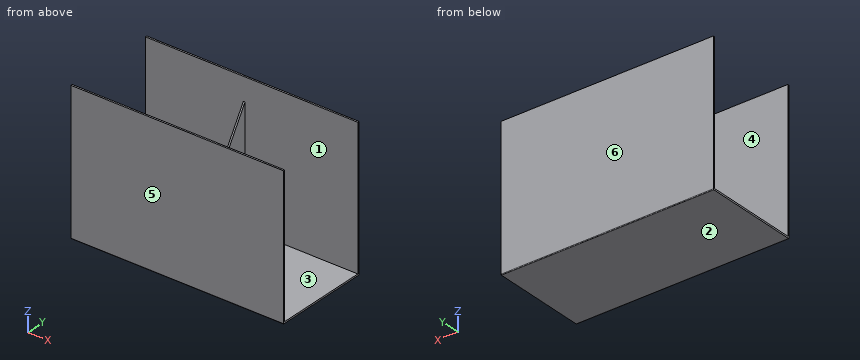
from build123d import *

# Parameters (mm, degrees)
F1_DEPTH = 650
F4_DEPTH = 5
F5_R     = 2


# Not quite as in the source:
# - a feature names something its author has since deleted; it is built from what else it names


with BuildPart() as f1:
    # F0 (on Right) → F1 (new body)
    with BuildSketch(Plane.YZ):
        Polygon((-295, 0), (0, 0), (0, 430), (-5, 430), (-5, 5), (-290, 5), (-290, 430), (-295, 430), align=None)
    extrude(amount=F1_DEPTH)

    # F3 (on offset) → F4 (join)
    with BuildSketch(Plane.YZ.offset(300)):
        Polygon((-230, 0), (-5, 0), (-5, 360), align=None)
    extrude(amount=F4_DEPTH)

    # F5
    f5_edges = [f1.edges().sort_by_distance(p)[0] for p in [
        (325, 0, 0),
        (325, -295, 0),
    ]]
    fillet(f5_edges, radius=F5_R)


solid = f1.part
Geometry: final body of the model. Coordinates: model frame, mm. Face numbers are marked on the shaded views. A direction names the side the tool comes from. Give positions to 0.01 mm unless a question says otherwise; leave off trailing zeros. Write each loop counter-clockwise with the first axis right and the second up, starting at its lowest first coordinate (ties: lowest second). Pieces come first, ordered by that corner, then holes. Notation, with made-up numbers: (36.5, 27) - (60.5, 27) arc R35 cw to (60.5, 59) - close; hole circle Ø7 at (46, -3). An arc over 180 degrees is marked (long way). Return JSON: item names as keys, results as strings. Group by question number.
1) Section B-B on y = -141. Return the cut outline in (x, z), plus the area to 3 significant figures.
2) Section A-A on z = 114. Return the cut outline in (x, y).
3) Set-up query: the marked faces 1 and 2. Return all of +Z, -Z, +X, -X, +Y, -Y with unobstructed straight access to the full face (end or side cutting, diameter ignored); none if empty.
4) Section D-D on z = 390.5. Return the cut outline in (x, y), plus the area to 3 significant figures.
5) Line query: line 1 (Y direction, x = 587, z = 75); line 2 (X direction, y = -68, z = 71.5); line 3 (Z direction, x = 148, y = -201). Output: solid intervals per line, ascending.
6) First-contact query: P1, Ø4, axis at x = 184.5, y = -44.5, coming from the +Z side; P2, Ø10, axis at y = -80, z = 109, coming from the +X side; P3, Ø8, axis at y = -129.5, z = 49, coming from the -X side. Flat tips, straight axial feed; report the tip coordinate or a pass-through.
7) Section C-C on x = 477. Return the cut outline in (y, z).
8) Mould query, pull axis Y, two halves, no side actions, for the marked faces 3, 4, 5 and 6. Classes: released by +Y, released by -Y, zero draft, split by the parting line, or undercut.
Filled in:
{
 "1": {"outline": "(0, 0) - (650, 0) - (650, 5) - (305, 5) - (305, 142.4) - (300, 142.4) - (300, 5) - (0, 5) - close", "area": "3,940 mm^2"},
 "2": {"outline": "(0, -295) - (650, -295) - (650, -290) - (0, -290) - close; (0, -5) - (300, -5) - (300, -158.75) - (305, -158.75) - (305, -5) - (650, -5) - (650, 0) - (0, 0) - close"},
 "3": {"face 1": "+Z", "face 2": "-Z, +X, -X, +Y, -Y"},
 "4": {"outline": "(0, -295) - (650, -295) - (650, -290) - (0, -290) - close; (0, -5) - (650, -5) - (650, 0) - (0, 0) - close", "area": "6,500 mm^2"},
 "5": {"line 1": "y = -295 to -290, -5 to 0", "line 2": "x = 300 to 305", "line 3": "z = 0 to 5"},
 "6": {"P1": "stops at z = 5", "P2": "stops at x = 305", "P3": "stops at x = 300"},
 "7": {"outline": "(-295, 2) arc R2 ccw to (-293, 0) - (-2, 0) arc R2 ccw to (0, 2) - (0, 430) - (-5, 430) - (-5, 5) - (-290, 5) - (-290, 430) - (-295, 430) - close"},
 "8": {"face 3": "undercut", "face 4": "undercut", "face 5": "released by -Y", "face 6": "released by +Y"}
}
